```python
from build123d import *

# Parameters (mm, degrees)
SKETCH1_R           = 14.2875
SKETCH1_R_2         = 1.6002
SKETCH1_R_3         = 2.4892
BOSS_EXTRUDE3_DEPTH = 3.175
SKETCH2_W           = 355.6
SKETCH2_H           = 19.05
CUT_EXTRUDE1_DEPTH  = 290.621961572
FILLET1_R           = 19.05
CUT_EXTRUDE2_DEPTH  = 290.621961572
FILLET2_R           = 6.35


with BuildPart() as part:
    # Sketch1 → Boss-Extrude3 (new body)
    with BuildSketch(Plane.XY):
        with BuildLine():
            Line((120.65, -152.4), (120.65, -6.35))
            Line((120.65, -6.35), (120.65, 6.35))
            ThreePointArc((120.65, 6.35), (124.369743879, 15.330256121), (133.35, 19.05))
            Line((133.35, 19.05), (165.1, 19.05))
            ThreePointArc((165.1, 19.05), (174.080256121, 15.330256121), (177.8, 6.35))
            Line((177.8, 6.35), (177.8, -6.35))
            Line((177.8, -6.35), (177.8, -222.25))
            ThreePointArc((177.8, -222.25), (175.940128061, -226.740128061), (171.45, -228.6))
            Line((171.45, -228.6), (12.7, -228.6))
            Line((12.7, -228.6), (-12.7, -228.6))
            Line((-12.7, -228.6), (-171.45, -228.6))
            ThreePointArc((-171.45, -228.6), (-175.940128061, -226.740128061), (-177.8, -222.25))
            Line((-177.8, -222.25), (-177.8, -6.35))
            Line((-177.8, -6.35), (-177.8, 6.35))
            ThreePointArc((-177.8, 6.35), (-174.080256121, 15.330256121), (-165.1, 19.05))
            Line((-165.1, 19.05), (-133.35, 19.05))
            ThreePointArc((-133.35, 19.05), (-124.369743879, 15.330256121), (-120.65, 6.35))
            Line((-120.65, 6.35), (-120.65, -6.35))
            Line((-120.65, -6.35), (-120.65, -152.4))
            ThreePointArc((-120.65, -152.4), (-113.210512242, -170.360512242), (-95.25, -177.8))
            Line((-95.25, -177.8), (-12.7, -177.8))
            Line((-12.7, -177.8), (12.7, -177.8))
            Line((12.7, -177.8), (95.25, -177.8))
            ThreePointArc((95.25, -177.8), (113.210512242, -170.360512242), (120.65, -152.4))
        make_face()
        with Locations((141.605, -25.4)):
            Circle(SKETCH1_R, mode=Mode.SUBTRACT)
        with Locations(Location((-141.605, -25.4, 0), (0, 0, 180))):
            Circle(SKETCH1_R, mode=Mode.SUBTRACT)
        with Locations((-141.605, -203.2)):
            Circle(SKETCH1_R, mode=Mode.SUBTRACT)
        with Locations((-141.605, -184.724802)):
            Circle(SKETCH1_R_2, mode=Mode.SUBTRACT)
        with Locations((-125.604004596, -193.962981004)):
            Circle(SKETCH1_R_2, mode=Mode.SUBTRACT)
        with Locations((-125.604004596, -212.439339011)):
            Circle(SKETCH1_R_2, mode=Mode.SUBTRACT)
        with Locations((-141.605, -221.677518015)):
            Circle(SKETCH1_R_2, mode=Mode.SUBTRACT)
        with Locations((-157.605995404, -212.439339011)):
            Circle(SKETCH1_R_2, mode=Mode.SUBTRACT)
        with Locations((-157.605995404, -193.962981004)):
            Circle(SKETCH1_R_2, mode=Mode.SUBTRACT)
        with Locations(Location((157.605995404, -212.439339011, 0), (0, 0, 180))):
            Circle(SKETCH1_R_2, mode=Mode.SUBTRACT)
        with Locations(Location((157.605995404, -193.962981004, 0), (0, 0, 180))):
            Circle(SKETCH1_R_2, mode=Mode.SUBTRACT)
        with Locations(Location((141.605, -184.724802, 0), (0, 0, 180))):
            Circle(SKETCH1_R_2, mode=Mode.SUBTRACT)
        with Locations(Location((125.604004596, -193.962981004, 0), (0, 0, 180))):
            Circle(SKETCH1_R_2, mode=Mode.SUBTRACT)
        with Locations(Location((125.604004596, -212.439339011, 0), (0, 0, 180))):
            Circle(SKETCH1_R_2, mode=Mode.SUBTRACT)
        with Locations(Location((141.605, -221.677518015, 0), (0, 0, 180))):
            Circle(SKETCH1_R_2, mode=Mode.SUBTRACT)
        with Locations(Location((141.605, -203.2, 0), (0, 0, 180))):
            Circle(SKETCH1_R, mode=Mode.SUBTRACT)
        with Locations((-76.2, -203.2)):
            Circle(SKETCH1_R_3, mode=Mode.SUBTRACT)
        with Locations(Location((76.2, -203.2, 0), (0, 0, 180))):
            Circle(SKETCH1_R_3, mode=Mode.SUBTRACT)
        with Locations((-25.4, -203.2)):
            Circle(SKETCH1_R_3, mode=Mode.SUBTRACT)
        with Locations((-127, -171.45)):
            Circle(SKETCH1_R_3, mode=Mode.SUBTRACT)
        with Locations((-149.225, 6.35)):
            Circle(SKETCH1_R_3, mode=Mode.SUBTRACT)
        with Locations(Location((127, -171.45, 0), (0, 0, 180))):
            Circle(SKETCH1_R_3, mode=Mode.SUBTRACT)
        with Locations(Location((149.225, 6.35, 0), (0, 0, 180))):
            Circle(SKETCH1_R_3, mode=Mode.SUBTRACT)
        with Locations((-168.275, -209.55)):
            Circle(SKETCH1_R_3, mode=Mode.SUBTRACT)
        with Locations(Location((168.275, -209.55, 0), (0, 0, 180))):
            Circle(SKETCH1_R_3, mode=Mode.SUBTRACT)
        with Locations((-165.1, -76.2)):
            Circle(SKETCH1_R_3, mode=Mode.SUBTRACT)
        with Locations(Location((165.1, -76.2, 0), (0, 0, 180))):
            Circle(SKETCH1_R_3, mode=Mode.SUBTRACT)
        with Locations(Location((25.4, -203.2, 0), (0, 0, 180))):
            Circle(SKETCH1_R_3, mode=Mode.SUBTRACT)
    extrude(amount=BOSS_EXTRUDE3_DEPTH)

    # Sketch2 → Cut-Extrude1 (cut, through all)
    with BuildSketch(Plane.XY.offset(3.175)):
        with Locations((0, 9.525)):
            Rectangle(SKETCH2_W, SKETCH2_H)
    extrude(amount=-CUT_EXTRUDE1_DEPTH, mode=Mode.SUBTRACT)

    # Fillet1
    fillet1_edges = [part.edges().sort_by_distance(p)[0] for p in [
        (-177.8, 0, 1.5875),
        (120.65, 0, 1.5875),
        (177.8, 0, 1.5875),
        (-120.65, 0, 1.5875),
    ]]
    fillet(fillet1_edges, radius=FILLET1_R)

    # Sketch3 → Cut-Extrude2 (cut, through all)
    with BuildSketch(Plane.XY.offset(3.175)):
        with BuildLine():
            ThreePointArc((-177.8, -19.05), (-172.220384182, -5.579615818), (-158.75, 0))
            Line((-158.75, 0), (-177.8, 0))
            Line((-177.8, 0), (-177.8, -19.05))
        make_face()
        with BuildLine():
            Line((-167.076337323, -57.15), (-167.076337323, -25.4))
            ThreePointArc((-167.076337323, -25.4), (-160.277331437, -8.075651132), (-143.51, 0))
            Line((-143.51, 0), (-158.75, 0))
            ThreePointArc((-158.75, 0), (-172.220384182, -5.579615818), (-177.8, -19.05))
            Line((-177.8, -19.05), (-177.8, -63.5))
            Line((-177.8, -63.5), (-173.426337323, -63.5))
            ThreePointArc((-173.426337323, -63.5), (-168.936209262, -61.640128061), (-167.076337323, -57.15))
        make_face()
    cut_extrude2 = extrude(amount=-CUT_EXTRUDE2_DEPTH, mode=Mode.SUBTRACT)

    # Mirror1: Cut-Extrude2 across plane
    add(cut_extrude2.mirror(Plane(origin=(0, 0, 0), x_dir=(0, 0, 1), z_dir=(1, 0, 0))), mode=Mode.SUBTRACT)

    # Fillet2
    fillet2_edges = [part.edges().sort_by_distance(p)[0] for p in [
        (177.8, -63.5, 1.5875),
        (-177.8, -63.5, 1.5875),
    ]]
    fillet(fillet2_edges, radius=FILLET2_R)


solid = part.part
```
The model under review builds one solid part; all positions refer to its coordinate system, in mm. A direction names the side the tool comes from. Give positions to 0.01 mm unless a question says otherwise; leave off trailing zeros. Write each loop counter-clockwise with the first axis right and the second up, starting at its lowest first coordinate (ties: lowest second). Pieces come first, ordered by that corner, then holes.
(1) Consider section B-B, the plane x = -150. Give the boundary of the cut face in (y, z) (3 decimals).
(2) Tool access review of faces 5 (the flat face through (2, -189, 0)), 6 (the cylindrical face through (113.01, -170.56, 1.57)): name each direction out of +Z, -Z, +X, -X, +Y, -Y from which nothing blocks a thin tool from reaching the whole face with its end or side.
(3) Consider section A-A, the plane y = -128.5. Give the boundary of the cut face in (x, z) (3 decimals).
(4) The part is to be moulded in two halves that separate along X. For faces 1 (the cylindrical face through (126.08, -5.73, 1.61)), 2 (the flat face through (2, -189, 3.175)), 3 (the cylindrical face through (160.458, -8.272, 1.61)), 4 (the cylindrical face through (-143.465, -189.034, 1.565)), say which applies: released by +X, released by -X, zero draft, split by the parting line, or undercut.
(5) Consider section D-D, the plane x = -41.5. Give the boundary of the cut face in (y, z) (3 decimals), and give its area (3 significant figures).
(6) To check wall thickness, follow L1, parallel to X at y = -143, z = 1.15; L2, parallel to X at y = -171.45, z = 2.1. State the ranges of each line that lie inside material, in increasing order.
(7) Consider section C-C, the plane z = 0.75. Give the number of separate pieces and of enclosed holes in the cut face, and give its area (3 significant figures).
(8) For P1, Ø4.5, axis at x = 165.1, y = -76.2, coming from the +Z side, flat-tipped, find the tip position at first contact; note if it passes through.
Returned:
1. outline: (-228.6, 0) - (-214.761, 0) - (-214.761, 3.175) - (-228.6, 3.175) - close; (-191.639, 0) - (-36.961, 0) - (-36.961, 3.175) - (-191.639, 3.175) - close; (-13.839, 0) - (-1.352, 0) - (-1.352, 3.175) - (-13.839, 3.175) - close
2. face 5: -Z, +X, -X, +Y, -Y
2. face 6: +Z, -Z, +Y
3. outline: (-177.8, 0) - (-120.65, 0) - (-120.65, 3.175) - (-177.8, 3.175) - close; (120.65, 0) - (177.8, 0) - (177.8, 3.175) - (120.65, 3.175) - close
4. face 1: undercut
4. face 2: zero draft
4. face 3: released by +X
4. face 4: undercut
5. outline: (-228.6, 0) - (-177.8, 0) - (-177.8, 3.175) - (-228.6, 3.175) - close
5. area: 161 mm2
6. L1: x = -177.8 to -120.65, 120.65 to 177.8
6. L2: x = -177.8 to -129.49, -124.51 to -112.05, 112.05 to 124.51, 129.49 to 177.8
7. separate pieces: 1
7. enclosed holes: 26
7. area: 34,000 mm2
8. P1: passes through
